Work out the finished part from the listing and answer in its coordinate system (mm). Face numbers are marked on the shaded views. A direction names the side the tool comes from. Round coordinates to 2 decimals unless told otherwise and drop trailing zeros. Write each loop counter-clockwise with the first axis right and the second up, starting at its lowest first coordinate (ties: lowest second). Pieces come first, ordered by that corner, then holes. Notation, with made-up numbers: (29, 34) -> (39, 34) arc R15 ccw to (39, 51) -> close; hole circle Ø5 at (-36, 37). An arc over 180 degrees is marked (long way). One line per item, written item: value.
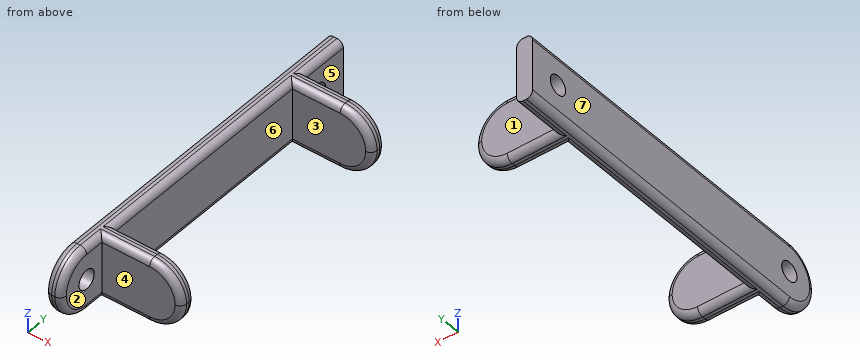
```python
from build123d import *

# Parameters (mm, degrees)
BOSS_EXTRUDE1_DEPTH = 20
SKETCH2_R           = 3
CUT_EXTRUDE1_DEPTH  = 20
FILLET1_R           = 10
FILLET2_R           = 2
CUT_EXTRUDE2_DEPTH  = 10


with BuildPart() as part:
    # Sketch1 → Boss-Extrude1 (new body)
    with BuildSketch(Plane.XY):
        Polygon((0, 0), (5, 0), (5, 10), (5, 16), (30, 16), (30, 21), (5, 21), (5, 91), (30, 91), (30, 96), (5, 96), (5, 170), (0, 170), align=None)
    extrude(amount=BOSS_EXTRUDE1_DEPTH)

    # Sketch2 → Cut-Extrude1 (cut)
    with BuildSketch(Plane.ZY):
        with Locations((10, 10)):
            Circle(SKETCH2_R)
        with Locations((10, 101.100788163)):
            Circle(SKETCH2_R)
    extrude(amount=-CUT_EXTRUDE1_DEPTH, mode=Mode.SUBTRACT)

    # Fillet1
    fillet1_edges = [part.edges().sort_by_distance(p)[0] for p in [
        (2.5, 170, 20),
        (2.5, 170, 0),
        (2.5, 0, 0),
        (2.5, 0, 20),
        (30, 18.5, 20),
        (30, 18.5, 0),
        (30, 93.5, 0),
        (30, 93.5, 20),
    ]]
    fillet(fillet1_edges, radius=FILLET1_R - 0.0001)  # a hair under: the kernel refuses the full size

    # Fillet2
    fillet2_edges = [part.edges().sort_by_distance(p)[0] for p in [
        (5, 56, 0),
        (12.50005, 16, 0),
        (12.50005, 96, 20),
        (5, 128.00005, 0),
        (12.50005, 96, 0),
        (12.50005, 91, 0),
        (5, 128.00005, 20),
        (12.50005, 16, 20),
        (5, 167.071097101, 2.928902899),
        (5, 167.071097101, 17.071097101),
        (0, 85, 20),
        (5, 12.99995, 20),
        (12.50005, 21, 20),
        (0, 85, 0),
        (0, 2.928902899, 17.071097101),
        (0, 2.928902899, 2.928902899),
        (0, 167.071097101, 2.928902899),
        (0, 167.071097101, 17.071097101),
        (12.50005, 91, 20),
        (12.50005, 21, 0),
        (5, 12.99995, 0),
        (5, 2.928902899, 17.071097101),
        (5, 56, 20),
        (5, 2.928902899, 2.928902899),
        (27.071097101, 21, 2.928902899),
        (27.071097101, 21, 17.071097101),
        (27.071097101, 16, 2.928902899),
        (27.071097101, 16, 17.071097101),
        (27.071097101, 96, 17.071097101),
        (27.071097101, 96, 2.928902899),
        (27.071097101, 91, 17.071097101),
        (27.071097101, 91, 2.928902899),
    ]]
    fillet(fillet2_edges, radius=FILLET2_R)

    # Sketch3 → Cut-Extrude2 (cut)
    with BuildSketch(Plane(origin=(5, 0, 0), x_dir=(0, 0, -1), z_dir=(1, 0, 0))):
        with BuildLine():
            Line((-2, 111.064309568), (0, 111.064309568))
            Line((0, 111.064309568), (5.411818178, 111.064309568))
            Line((5.411818178, 111.064309568), (5.411818178, 180.556551252))
            Line((5.411818178, 180.556551252), (-29.02399195, 180.556551252))
            Line((-29.02399195, 180.556551252), (-29.02399195, 111.064309568))
            Line((-29.02399195, 111.064309568), (-20, 111.064309568))
            Line((-20, 111.064309568), (-18, 111.064309568))
            Line((-18, 111.064309568), (-18, 160))
            ThreePointArc((-18, 160), (-15.656854249, 165.656854249), (-10, 168))
            ThreePointArc((-10, 168), (-4.343145751, 165.656854249), (-2, 160))
            Line((-2, 160), (-2, 111.064309568))
        make_face()
        with BuildLine():
            Line((-18, 111.064309568), (-2, 111.064309568))
            Line((-2, 111.064309568), (-2, 160))
            ThreePointArc((-2, 160), (-4.343145751, 165.656854249), (-10, 168))
            ThreePointArc((-10, 168), (-15.656854249, 165.656854249), (-18, 160))
            Line((-18, 160), (-18, 111.064309568))
        make_face()
    extrude(amount=-CUT_EXTRUDE2_DEPTH, mode=Mode.SUBTRACT)


solid = part.part
```
(1) Flat-ended cylindrical pins translate along their axes: pin 1 Ø4.5 at (y, z) = (104, 13.5) entering from +X; pin 2 Ø8 at (x, z) = (21, 9) entering from +Y; pin 3 Ø1 at (x, z) = (4, 6.5) entering from -Y; pin 4 Ø8 at (y, z) = (10, 10) entering from -X. Find the tip coordinate at first contact, or state that the pin passes through.
Reported:
pin 1: stops at x = 5
pin 2: stops at y = 96
pin 3: stops at y = 0.62
pin 4: stops at x = 0
(2) Find section B-B on y = 48.5. Give the vertices of the cut face in (x, z), plus the area to 3 significant figures.
Reported:
outline: (0, 2) arc R2 ccw to (2, 0) -> (3, 0) arc R2 ccw to (5, 2) -> (5, 18) arc R2 ccw to (3, 20) -> (2, 20) arc R2 ccw to (0, 18) -> close
area: 96.6 mm2
(3) A tool of negligible diameter and unlimited length cuts with its end or side. For the marked faces 5, 6 and 7, from which of +Z, -Z, +X, -X, +Y, -Y can it reach the whole face along a straight path? Write none if from no direction.
Reported:
face 5: +Z, -Z, +X, +Y
face 6: +Z, -Z, +X
face 7: +Z, -Z, -X, +Y, -Y
(4) Find section A-A on x = 17.5. Give the vertices of the cut face in (y, z).
Reported:
outline: (16, 2) arc R2 ccw to (18, 0) -> (19, 0) arc R2 ccw to (21, 2) -> (21, 18) arc R2 ccw to (19, 20) -> (18, 20) arc R2 ccw to (16, 18) -> close; (91, 2) arc R2 ccw to (93, 0) -> (94, 0) arc R2 ccw to (96, 2) -> (96, 18) arc R2 ccw to (94, 20) -> (93, 20) arc R2 ccw to (91, 18) -> close
(5) For a pull along Y with two mould halves and no side action, classify the marked faces 1, 2, 3 and 4 as pulls with the +Y half, pulls with the -Y half, needs draft (parallel to the pull), parting line crosses it, or undercut.
Reported:
face 1: pulls with the +Y half
face 2: needs draft
face 3: undercut
face 4: pulls with the -Y half
(6) Consider probe 1 along Y at (x, z) = (2.95, 10); probe 2 along Y at (x, z) = (6, 15.75); probe 3 along Y at (x, z) = (3.9, 10). Determine where each line is inside the solid, lowest interval first.
Reported:
probe 1: y = 0 to 7, 13 to 98.1, 104.1 to 111.06
probe 2: y = 16 to 21, 91 to 96
probe 3: y = 0.21 to 7, 13 to 98.1, 104.1 to 111.06
